from build123d import *
from build123d.topology import SkipClean

# Parameters (mm, degrees)
ESBO_O1_R                = 11.15
RESSALTO_EXTRUS_O1_DEPTH = 15
ESBO_O2_R                = 22.5
RESSALTO_EXTRUS_O2_DEPTH = 4
RESSALTO_EXTRUS_O6_START = -8
ESBO_O5_R                = 11.15
ESBO_O5_R_2              = 8
RESSALTO_EXTRUS_O6_DEPTH = 8
RESSALTO_EXTRUS_O7_START = 4
ESBO_O7_R                = 14.2
ESBO_O7_R_2              = 11.15
RESSALTO_EXTRUS_O7_DEPTH = 4
RESSALTO_EXTRUS_O8_START = 4
ESBO_O8_R                = 11.15
ESBO_O8_R_2              = 8
RESSALTO_EXTRUS_O8_DEPTH = 4
CORTE_EXTRUS_O1_DEPTH    = 7


with BuildPart() as part:
    # Esbo_o1 → Ressalto-extrus_o1 (new body)
    with BuildSketch(Plane.XY):
        with BuildLine():
            Line((-2.5, 18), (-2.5, 13.978197309))
            ThreePointArc((-2.5, 13.978197309), (-10.040916293, 10.040916293), (-13.978197309, 2.5))
            Line((-13.978197309, 2.5), (-18, 2.5))
            Line((-18, 2.5), (-18, -2.5))
            Line((-18, -2.5), (-13.978197309, -2.5))
            ThreePointArc((-13.978197309, -2.5), (-10.040916293, -10.040916293), (-2.5, -13.978197309))
            Line((-2.5, -13.978197309), (-2.5, -18))
            Line((-2.5, -18), (2.5, -18))
            Line((2.5, -18), (2.5, -13.978197309))
            ThreePointArc((2.5, -13.978197309), (10.040916293, -10.040916293), (13.978197309, -2.5))
            Line((13.978197309, -2.5), (18, -2.5))
            Line((18, -2.5), (18, 2.5))
            Line((18, 2.5), (13.978197309, 2.5))
            ThreePointArc((13.978197309, 2.5), (10.040916293, 10.040916293), (2.5, 13.978197309))
            Line((2.5, 13.978197309), (2.5, 18))
            Line((2.5, 18), (-2.5, 18))
        make_face()
        Circle(ESBO_O1_R, mode=Mode.SUBTRACT)
    extrude(amount=RESSALTO_EXTRUS_O1_DEPTH)

    # Esbo_o5 → Ressalto-extrus_o6 (add)
    with BuildSketch(Plane.XY.offset(15).offset(RESSALTO_EXTRUS_O6_START)):
        Circle(ESBO_O5_R)
        Circle(ESBO_O5_R_2, mode=Mode.SUBTRACT)
    extrude(amount=RESSALTO_EXTRUS_O6_DEPTH)



with BuildPart() as body_2:
    # Esbo_o2 → Ressalto-extrus_o2 (new body)
    # profile 1 of 5: a face of its own
    with SkipClean():  # the faces are left unmerged after this step: merging them gives an invalid solid
        with BuildSketch(Plane(origin=(0, 0, 0), x_dir=(-1, 0, 0), z_dir=(0, 0, -1))):
            Circle(ESBO_O2_R)
            with BuildLine():
                Line((2.5, 13.978197309), (2.5, 18))
                Line((2.5, 18), (-2.5, 18))
                Line((-2.5, 18), (-2.5, 13.978197309))
                ThreePointArc((-2.5, 13.978197309), (-10.040916293, 10.040916293), (-13.978197309, 2.5))
                Line((-13.978197309, 2.5), (-18, 2.5))
                Line((-18, 2.5), (-18, -2.5))
                Line((-18, -2.5), (-13.978197309, -2.5))
                ThreePointArc((-13.978197309, -2.5), (-10.040916293, -10.040916293), (-2.5, -13.978197309))
                Line((-2.5, -13.978197309), (-2.5, -18))
                Line((-2.5, -18), (2.5, -18))
                Line((2.5, -18), (2.5, -13.978197309))
                ThreePointArc((2.5, -13.978197309), (10.040916293, -10.040916293), (13.978197309, -2.5))
                Line((13.978197309, -2.5), (18, -2.5))
                Line((18, -2.5), (18, 2.5))
                Line((18, 2.5), (13.978197309, 2.5))
                ThreePointArc((13.978197309, 2.5), (10.040916293, 10.040916293), (2.5, 13.978197309))
            make_face(mode=Mode.SUBTRACT)
        # profile 2 of 5: a face of its own
        with BuildSketch(Plane(origin=(0, 0, 0), x_dir=(-1, 0, 0), z_dir=(0, 0, -1))):
            with BuildLine():
                Line((2.5, -18), (2.5, -13.978197309))
                ThreePointArc((2.5, -13.978197309), (0, -14.2), (-2.5, -13.978197309))
                Line((-2.5, -13.978197309), (-2.5, -18))
                Line((-2.5, -18), (2.5, -18))
            make_face()
        # profile 3 of 5: a face of its own
        with BuildSketch(Plane(origin=(0, 0, 0), x_dir=(-1, 0, 0), z_dir=(0, 0, -1))):
            with BuildLine():
                ThreePointArc((-13.978197309, -2.5), (-14.2, 0), (-13.978197309, 2.5))
                Line((-13.978197309, 2.5), (-18, 2.5))
                Line((-18, 2.5), (-18, -2.5))
                Line((-18, -2.5), (-13.978197309, -2.5))
            make_face()
        # profile 4 of 5: a face of its own
        with BuildSketch(Plane(origin=(0, 0, 0), x_dir=(-1, 0, 0), z_dir=(0, 0, -1))):
            with BuildLine():
                ThreePointArc((-2.5, 13.978197309), (0, 14.2), (2.5, 13.978197309))
                Line((2.5, 13.978197309), (2.5, 18))
                Line((2.5, 18), (-2.5, 18))
                Line((-2.5, 18), (-2.5, 13.978197309))
            make_face()
        # profile 5 of 5: a face of its own
        with BuildSketch(Plane(origin=(0, 0, 0), x_dir=(-1, 0, 0), z_dir=(0, 0, -1))):
            with BuildLine():
                Line((18, 2.5), (13.978197309, 2.5))
                ThreePointArc((13.978197309, 2.5), (14.2, 0), (13.978197309, -2.5))
                Line((13.978197309, -2.5), (18, -2.5))
                Line((18, -2.5), (18, 2.5))
            make_face()
        extrude(amount=RESSALTO_EXTRUS_O2_DEPTH)


with BuildPart() as part_1:
    with SkipClean():  # the faces are left unmerged after this step: merging them gives an invalid solid
        add(part.part)

        add(body_2.part)  # Ressalto-extrus_o7 merges body 2
        # Esbo_o7 → Ressalto-extrus_o7 (add)
        with BuildSketch(Plane(origin=(0, 0, 0), x_dir=(-1, 0, 0), z_dir=(0, 0, -1)).offset(RESSALTO_EXTRUS_O7_START)):
            Circle(ESBO_O7_R)
            with Locations(Location((0, 0, 0), (0, 0, 180))):
                Circle(ESBO_O7_R_2, mode=Mode.SUBTRACT)
        extrude(amount=-RESSALTO_EXTRUS_O7_DEPTH)

    # Esbo_o8 → Ressalto-extrus_o8 (add)
    with BuildSketch(Plane(origin=(0, 0, 7), x_dir=(-1, 0, 0), z_dir=(0, 0, -1)).offset(RESSALTO_EXTRUS_O8_START)):
        Circle(ESBO_O8_R)
        with Locations(Location((0, 0, 0), (0, 0, 180))):
            Circle(ESBO_O8_R_2, mode=Mode.SUBTRACT)
    extrude(amount=-RESSALTO_EXTRUS_O8_DEPTH)

    # Esbo_o11 → Corte-extrus_o1 (cut)
    with BuildSketch(Plane.XY.offset(15)):
        with BuildLine():
            Line((-11.191152491, -5.789482353), (-8.437773704, -4.365085901))
            ThreePointArc((-8.437773704, -4.365085901), (0.195118203, -9.497996046), (8.609923977, -4.014873487))
            Line((8.609923977, -4.014873487), (11.419478117, -5.324990098))
            ThreePointArc((11.419478117, -5.324990098), (0.258788353, -12.597342124), (-11.191152491, -5.789482353))
        make_face()
        with BuildLine():
            Line((-11.419478117, 5.324990098), (-8.609923977, 4.014873487))
            ThreePointArc((-8.609923977, 4.014873487), (-0.195118203, 9.497996046), (8.437773704, 4.365085901))
            Line((8.437773704, 4.365085901), (11.191152491, 5.789482353))
            ThreePointArc((11.191152491, 5.789482353), (-0.258788353, 12.597342124), (-11.419478117, 5.324990098))
        make_face()
    extrude(amount=-CORTE_EXTRUS_O1_DEPTH, mode=Mode.SUBTRACT)


solid = part_1.part
Source: CAD feature listing. Evaluate the final solid. Frame: model axes, mm. A direction names the side the tool comes from. Coordinates: 2 decimals unless noted, no trailing zeros. Loops run counter-clockwise (first coordinate to the right, second up) from the corner with the lowest first, then second, coordinate; pieces in that order, holes last. Notation, with made-up numbers: (-7.5, 38.5) - (-2.5, 38.5) arc R19 cw to (-2.5, 70.5) - close; hole circle Ø6 at (42, 61.25). An arc over 180 degrees is marked (long way). One line per item, written item: value. Start each with the question number.
1. Contact query for flat-ended pins moving along their axis: P1, Ø3, axis at y = -16.5, z = 8, coming from the -X side; P2, Ø2, axis at x = -9, z = 10.5, coming from the +Y side; P3, Ø4, axis at y = -0.5, z = 11.5, coming from the +X side; P4, Ø18.5, axis at x = 0, y = 0, coming from the +Z side. Output: stop coordinate, or through.
2. Set-up query: faces 1 (the flat face through (-16, -2.5, 7)), 2 (the cylindrical face through (10.126, 9.955, 7.395)), 3 (the flat face through (-16, 2.5, 7)), 4 (the flat face through (-5, -15, 0)). Return all of +Z, -Z, +X, -X, +Y, -Y with unobstructed straight access to the full face (end or side cutting, diameter ignored); none if empty.
3. Section D-D (z = 2). Return the cut outline in (x, y).
4. Section B-B (y = 0). Return the cut outline in (x, z), and give its area (3 significant figures).
5. Ray query, L1, parallel to Y at x = 0, z = 8.75; L2, parallel to Y at x = 0, z = -3.1; L3, parallel to Z at x = 6.5, y = 13.5. Return the intervals inside material, ascending.
6. Section A-A (x = 0). Return the cut outline in (y, z).
7. Mould query, pull axis Y, two halves, no side actions, for faces 5 (the flat face through (0, 18, 7)), 6 (the flat face through (3, 8, 3)), 7 (the cylindrical face through (9.955, -10.126, 7.395)), 8 (the flat face through (2.5, -16, 7)). Classes: pulls with the +Y half, pulls with the -Y half, needs draft (parallel to the pull), parting line crosses it, or undercut.
8. Section C-C (z = 10.25). Return the cut outline in (x, y) (3 decimals).
Verdict:
1. P1: stops at x = -2.5
1. P2: stops at y = 11.73
1. P3: stops at x = 18
1. P4: stops at z = 15
2. face 1: +Z, -X, -Y
2. face 2: +Z, +X, +Y
2. face 3: +Z, -X, +Y
2. face 4: +Z
3. outline: (-18, -2.5) - (-13.98, -2.5) arc R14.2 ccw to (-2.5, -13.98) - (-2.5, -18) - (2.5, -18) - (2.5, -13.98) arc R14.2 ccw to (13.98, -2.5) - (18, -2.5) - (18, 2.5) - (13.98, 2.5) arc R14.2 ccw to (2.5, 13.98) - (2.5, 18) - (-2.5, 18) - (-2.5, 13.98) arc R14.2 ccw to (-13.98, 2.5) - (-18, 2.5) - close; hole circle Ø22.3 at (0, 0)
4. outline: (-22.5, -4) - (-11.15, -4) - (-11.15, 3) - (-8, 3) - (-8, 15) - (-18, 15) - (-18, 0) - (-22.5, 0) - close; (8, 3) - (11.15, 3) - (11.15, -4) - (22.5, -4) - (22.5, 0) - (18, 0) - (18, 15) - (8, 15) - close
4. area: 372 mm2
5. L1: y = -18 to -12.6, -9.5 to -8, 8 to 9.5, 12.6 to 18
5. L2: y = -22.5 to -11.15, 11.15 to 22.5
5. L3: z = -4 to 0
6. outline: (-22.5, -4) - (-11.15, -4) - (-11.15, 3) - (-8, 3) - (-8, 15) - (-9.5, 15) - (-9.5, 8) - (-12.6, 8) - (-12.6, 15) - (-18, 15) - (-18, 0) - (-22.5, 0) - close; (8, 3) - (11.15, 3) - (11.15, -4) - (22.5, -4) - (22.5, 0) - (18, 0) - (18, 15) - (12.6, 15) - (12.6, 8) - (9.5, 8) - (9.5, 15) - (8, 15) - close
7. face 5: pulls with the +Y half
7. face 6: undercut
7. face 7: pulls with the -Y half
7. face 8: needs draft
8. outline: (-18, -2.5) - (-13.978, -2.5) arc R14.2 ccw to (-2.5, -13.978) - (-2.5, -18) - (2.5, -18) - (2.5, -13.978) arc R14.2 ccw to (13.978, -2.5) - (18, -2.5) - (18, 2.5) - (13.978, 2.5) arc R14.2 ccw to (2.5, 13.978) - (2.5, 18) - (-2.5, 18) - (-2.5, 13.978) arc R14.2 ccw to (-13.978, 2.5) - (-18, 2.5) - close; hole (-11.419, 5.325) - (-8.61, 4.015) arc R9.5 cw to (8.438, 4.365) - (11.191, 5.789) arc R12.6 ccw to start; hole (-11.191, -5.789) arc R12.6 ccw to (11.419, -5.325) - (8.61, -4.015) arc R9.5 cw to (-8.438, -4.365) - close; hole circle Ø16 at (0, 0)
